Source: CAD feature listing. Evaluate the final solid. Frame: model axes, mm. Face numbers are marked on the shaded views. A direction names the side the tool comes from. Coordinates: 2 decimals unless noted, no trailing zeros. Loops run counter-clockwise (first coordinate to the right, second up) from the corner with the lowest first, then second, coordinate; pieces in that order, holes last.
Item 1: Section query A-A, the plane y = -17.5. Return the cut outline in (x, z).
Item 2: Section query C-C, the plane y = 17.5. Return the cut outline in (x, z), then the cut area to 3 significant figures.
Item 3: Line query: probe 1 along Y at (x, z) = (32, 0.8); probe 2 along Y at (x, z) = (-1.5, 5.75); probe 3 along Z at (x, y) = (18.5, -12.5). Output: solid intervals per line, ascending.
Item 4: Reachability of the marked faces 1 and 2 from +Z, -Z, +X, -X, +Y, -Y: full face, straight path, thin tool, end or side. Return the list, or none.
Item 5: Pin query (flat end, axial travel): pin 1 Ø4 at (y, z) = (17.5, 6) entering from -X; pin 2 Ø3 at (y, z) = (17, 6.5) entering from +X; pin 3 Ø1.8 at (x, y) = (-32, 17.5) entering from -Z; pin 4 Ø19.5 at (x, y) = (-14.5, -5) entering from +Z. Return the tip coordinate at first contact, or that it passes through.
Item 6: Section query D-D, the plane z = 7.25. Return the cut outline in (x, y).
Item 7: Section query B-B, the plane x = -32. Return the cut outline in (y, z), then the cut area to 3 significant figures.
Autodesk Inventor part; units mm, degrees
ref_plane "YZ Plane" through (0, 0, 0) normal (1, 0, 0) x (0, 1, 0)
ref_plane "XZ Plane" through (0, 0, 0) normal (0, 1, 0) x (-1, 0, 0)
ref_plane "XY Plane" through (0, 0, 0) normal (0, 0, 1) x (1, 0, 0)
sketch "스케치1" plane through (0, 0, 0) normal (0, 0, 1) x (1, 0, 0)
  line L0 (-34, 19.5) -> (34, 19.5)
  line L1 (34, 19.5) -> (34, -19.5)
  line L2 (34, -19.5) -> (-34, -19.5)
  line L3 (-34, -19.5) -> (-34, 19.5)
  line L4 (-34, 19.5) -> (34, -19.5) construction
  line L5 (34, 19.5) -> (-34, -19.5) construction
  point P0 (0, 0)
  dimension "d0" = 68
  dimension "d1" = 39
extrude "돌출1" add sketch "스케치1" along normal blind 1.6
sketch "스케치3" plane through (0, 0, 1.6) normal (0, 0, 1) x (1, 0, 0)
  circle A0 centre (32, 17.5) radius 2
  circle A1 centre (-32, 17.5) radius 2
  circle A2 centre (-32, -17.5) radius 2
  circle A3 centre (32, -17.5) radius 2
  line L0 (34, 19.5) -> (-34, 19.5)
  line L1 (34, -19.5) -> (34, 19.5)
  line L2 (-34, -19.5) -> (34, -19.5)
  line L3 (-34, 19.5) -> (-34, -19.5)
  circle A4 centre (-32, 17.5) radius 1.5
  circle A5 centre (32, 17.5) radius 1.5
  circle A6 centre (32, -17.5) radius 1.5
  circle A7 centre (-32, -17.5) radius 1.5
  point P0 (0, 0)
  dimension "d4" = 4
  dimension "d5" = 4
  dimension "d6" = 4
  dimension "d7" = 4
  dimension "d8" = 3
  dimension "d9" = 3
  dimension "d10" = 3
  dimension "d11" = 3
extrude "돌출2" cut sketch "스케치3" against normal up to surface (1.6 mm away) contours A4 | A5 | A6 | A7
sketch "스케치4" plane through (0, 0, 1.6) normal (0, 0, 1) x (1, 0, 0)
  line L0 (4, 15.9921) -> (-4, 15.9921)
  line L1 (-4, 15.9921) -> (-4, 19.5)
  line L2 (-4, 19.5) -> (4, 19.5)
  line L3 (4, 19.5) -> (4, 15.9921)
  line L4 (4, 15.9921) -> (-4, 19.5) construction
  line L5 (-4, 15.9921) -> (4, 19.5) construction
  line L6 (34, 19.5) -> (-34, 19.5)
  line L7 (0, -27.3) -> (0, 27.3)
  point P0 (0, 0)
  point P1 (0, 17.746)
  point P2 (0, 19.5)
  point P3 (-4, 17.746)
  dimension "d14" = 8
extrude "돌출3" add sketch "스케치4" along normal blind 12
properties part number "컨버터"
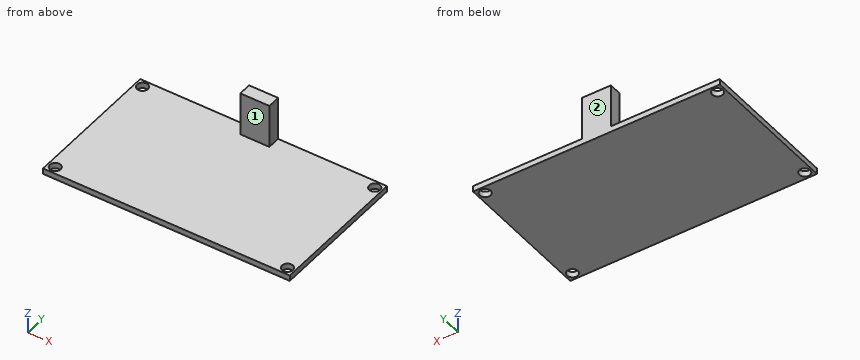
Verdict:
1. outline: (-34, 0) - (-33.5, 0) - (-33.5, 1.6) - (-34, 1.6) - close; (-30.5, 0) - (30.5, 0) - (30.5, 1.6) - (-30.5, 1.6) - close; (33.5, 0) - (34, 0) - (34, 1.6) - (33.5, 1.6) - close
2. outline: (-34, 0) - (-33.5, 0) - (-33.5, 1.6) - (-34, 1.6) - close; (-30.5, 0) - (30.5, 0) - (30.5, 1.6) - (4, 1.6) - (4, 13.6) - (-4, 13.6) - (-4, 1.6) - (-30.5, 1.6) - close; (33.5, 0) - (34, 0) - (34, 1.6) - (33.5, 1.6) - close
2. area: 195 mm2
3. probe 1: y = -19.5 to -19, -16 to 16, 19 to 19.5
3. probe 2: y = 15.99 to 19.5
3. probe 3: z = 0 to 1.6
4. face 1: +Z, +X, -X, -Y
4. face 2: +Z, -Z, +X, -X, +Y
5. pin 1: stops at x = -4
5. pin 2: stops at x = 4
5. pin 3: passes through
5. pin 4: stops at z = 1.6
6. outline: (-4, 15.99) - (4, 15.99) - (4, 19.5) - (-4, 19.5) - close
7. outline: (-19.5, 0) - (-19, 0) - (-19, 1.6) - (-19.5, 1.6) - close; (-16, 0) - (16, 0) - (16, 1.6) - (-16, 1.6) - close; (19, 0) - (19.5, 0) - (19.5, 1.6) - (19, 1.6) - close
7. area: 52.8 mm2
